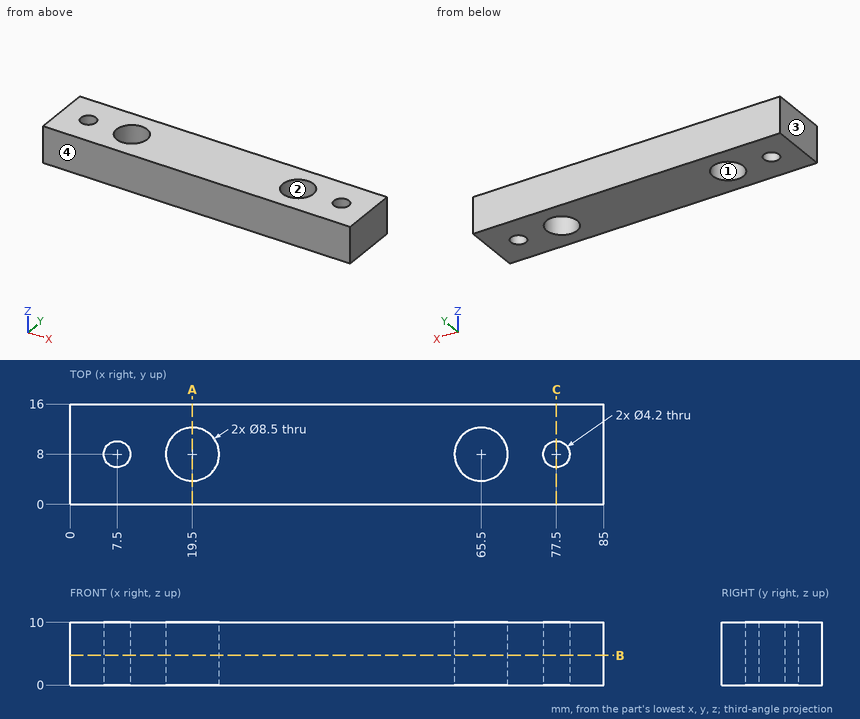
Part print with two shaded views. Sizes in mm from the minimum x, y, z corner. Round coordinates to 2 decimals unless told otherwise and drop trailing zeros. Loops run counter-clockwise (first coordinate to the right, second up) from the corner with the lowest first, then second, coordinate; pieces in that order, holes last. Notation, with made-up numbers: M -12.75,85 L 2.25,85 A30 cw 2.25,119 Z; hole C 63.5,41.25 d8. An arc over 180 degrees is marked long. Put each result on its own line as item: value. Start each with the question number.
Item 1: Cut at B-B (z = 4.75). List the corners of the cut face in (x, y), then the cut area to 3 significant figures.
Item 2: Drop a flat-ended pin along its axis: P1, Ø1, axis at y = 8.5, z = 3, coming from the -X side. Give the stop position or say it passes through.
Item 3: Mould opens along Y. For the marked faces 1, 2, 3 and 4 say: released by +Y, released by -Y, zero draft, split by the parting line, or undercut.
Item 4: Cut at A-A (x = 19.5). List the corners of the cut face in (y, z).
Item 5: Cut at C-C (x = 77.5). List the corners of the cut face in (y, z), then the cut area to 3 significant figures.
Item 6: Drill centre lines: line 1 along Y through (x, z) = (77.5, 6.75); line 2 along X through (y, z) = (5.25, 7); line 3 along Y through (x, z) = (19.5, 6.5). Where is each one in solid material? Low to high.
Answer block:
1. outline: M 0,0 L 85,0 L 85,16 L 0,16 Z; hole C 7.5,8 d4.2; hole C 19.5,8 d8.5; hole C 65.5,8 d8.5; hole C 77.5,8 d4.2
1. area: 1,220 mm2
2. P1: x = 0
3. face 1: undercut
3. face 2: undercut
3. face 3: zero draft
3. face 4: released by -Y
4. outline: M 0,0 L 3.75,0 L 3.75,10 L 0,10 Z; M 12.25,0 L 16,0 L 16,10 L 12.25,10 Z
5. outline: M 0,0 L 5.9,0 L 5.9,10 L 0,10 Z; M 10.1,0 L 16,0 L 16,10 L 10.1,10 Z
5. area: 118 mm2
6. line 1: 0 to 5.9, 10.1 to 16
6. line 2: 0 to 16.26, 22.74 to 62.26, 68.74 to 85
6. line 3: 0 to 3.75, 12.25 to 16
